Autodesk Inventor part; units mm, degrees
ref_plane "Work Plane1" through (-210, 0.3, -39.7) normal (1, 0, 0) x (0, 0, -1)
ref_plane "YZ Plane" through (0, 0, 0) normal (1, 0, 0) x (0, 1, 0)
ref_plane "XZ Plane" through (0, 0, 0) normal (0, 1, 0) x (-1, 0, 0)
sketch "Sketch1" plane through (0, 0, 0) normal (0, 1, 0) x (-1, 0, 0)
  line L0 (0, 0) -> (420, 0)
  line L1 (420, 0) -> (420, -40)
  line L2 (420, -40) -> (0, -40)
  line L3 (0, -40) -> (0, 0)
  dimension "d0" = 420
  dimension "d1" = 40
extrude "Extrusion1" add sketch "Sketch1" along normal blind 3.5
fillet "Fillet1" radius 0.3 10 edges at (-210, 3.5, 0) (-210, 0, 0) (0, 0, -20) (0, 3.5, -20) (0, 1.75, -40) (-210, 3.5, -40) (-210, 0, -40) (-420, 0, -20) (-420, 1.75, -40) (-420, 3.5, -20)
sketch "Sketch2" plane through (0, 0, 0) normal (0, -1, 0) x (1, 0, 0)
  line L0 (-419.7, -39.7) -> (-419.7, -0.3)
  line L1 (-419.7, -20) -> (0, -20)
  circle A0 centre (-405, -20) radius 5
  circle A1 centre (-375, -20) radius 5
  circle A2 centre (-345, -20) radius 5
  circle A3 centre (-315, -20) radius 5
  line L2 (-420, 0) -> (-420, -39.7)
  line L3 (-315, -20) -> (-315, -8.0411)
  line L4 (-210.3, -20) -> (-630, -20)
  circle A4 centre (-225, -20) radius 5
  circle A5 centre (-255, -20) radius 5
  circle A6 centre (-285, -20) radius 5
  point P0 (0, 0)
  point P1 (-420, -0.3)
  dimension "d5" = 10
  dimension "d6" = 10
  dimension "d7" = 10
  dimension "d8" = 10
  dimension "d9" = 15
  dimension "d10" = 30
  dimension "d11" = 30
  dimension "d12" = 30
ref_plane "Work Plane1" through (-210, 0.3, -39.7) normal (1, 0, 0) x (0, 0, -1)
extrude "Extrusion2" cut sketch "Sketch2" against normal blind 3
mirror "Mirror1" about plane through (-210, 0.3, -39.7) normal (1, 0, 0) of "Extrusion2"
fillet "Fillet2" radius 2 6 edges at (-0.0879, 3.4121, -0.0879) (-0.0879, 0.0879, -0.0879) (0, 1.75, 0) (-419.9121, 3.4121, -0.0879) (-419.9121, 0.0879, -0.0879) (-420, 1.75, 0)
sketch "Sketch3" plane through (0, 3.5, 0) normal (0, 1, 0) x (1, 0, 0)
  line L0 (4.2695, -58.2258) -> (-175.7305, -58.2258)
  line L1 (-175.7305, -58.2258) -> (-175.7305, 85.9661)
  line L2 (-175.7305, 85.9661) -> (4.2695, 85.9661)
  line L3 (4.2695, 85.9661) -> (4.2695, -58.2258)
  line L4 (-175.7305, 85.9661) -> (-355.7305, 85.9661)
  line L5 (-355.7305, 85.9661) -> (-355.7305, -58.2258)
  line L6 (-355.7305, -58.2258) -> (-175.7305, -58.2258)
  line L7 (-175.7305, -58.2258) -> (-175.7305, 85.9661)
  line L8 (-355.7305, -58.2258) -> (-453.8172, -58.2258)
  line L9 (-453.8172, -58.2258) -> (-453.8172, 85.9661)
  line L10 (-453.8172, 85.9661) -> (-355.7305, 85.9661)
  line L11 (-355.7305, 85.9661) -> (-355.7305, -58.2258)
  point P0 (0, 0)
  dimension "d18" = 180
  dimension "d19" = 180
extrude "Extrusion8" cut sketch "Sketch3" against normal through all contours L0 L1 L2 L3 | L6 L5 L4 L1
sketch "Sketch7" plane through (-355.7305, 3.5, -0.3) normal (1, 0, 0) x (0, 0, -1)
  line L0 (4.7, -1.75) -> (14.7, -1.75) construction
  line L1 (-0.3, -3.2) -> (-0.3, -0.3)
  line L2 (4.7, -2.5) -> (14.7, -2.5)
  line L3 (14.7, -1) -> (4.7, -1)
  arc A0 (4.7, -1) -> (4.7, -2.5) centre (4.7, -1.75) ccw
  arc A1 (14.7, -2.5) -> (14.7, -1) centre (14.7, -1.75) ccw
  line L4 (24.7, -1.75) -> (34.7, -1.75) construction
  line L5 (24.7, -2.5) -> (34.7, -2.5)
  line L6 (34.7, -1) -> (24.7, -1)
  arc A2 (24.7, -1) -> (24.7, -2.5) centre (24.7, -1.75) ccw
  arc A3 (34.7, -2.5) -> (34.7, -1) centre (34.7, -1.75) ccw
  line L7 (39.7, -0.3) -> (39.7, -3.2)
  point P0 (-0.3, -3.5)
  point P1 (9.7, -1.75)
  point P2 (29.7, -1.75)
  dimension "d56" = 5
  dimension "d57" = 1.5
  dimension "d58" = 5
  dimension "d59" = 1.5
  dimension "d60" = 10
  dimension "d61" = 10
extrude "Extrusion9" cut sketch "Sketch7" against normal blind 16
chamfer "Chamfer3" distance 0.3 angle 45 8 edges at (-355.7305, 2.5, -10) (-355.7305, 1.75, -15.75) (-355.7305, 1, -10) (-355.7305, 1.75, -4.25) (-355.7305, 1.75, -24.25) (-355.7305, 2.5, -30) (-355.7305, 1.75, -35.75) (-355.7305, 1, -30)
properties part number "LeftClamo3"
Read the model definition and answer for the solid it produces. Units are mm, in the model's axes. A direction names the side the tool comes from. Round coordinates to 2 decimals unless told otherwise and drop trailing zeros. Write each loop counter-clockwise with the first axis right and the second up, starting at its lowest first coordinate (ties: lowest second). Pieces come first, ordered by that corner, then holes. Notation, with made-up numbers: (4.5, 0.25) - (21.5, 0.25) arc R26 ccw to (21.5, 35.25) - close; hole circle Ø1 at (9.25, -37.75). An arc over 180 degrees is marked (long way). Use CSV: the item, a comma, the result in double quotes.
Q1. Each of these flat-tipped pins is pushed along its axis until it touches: pin 1 Ø3 at (x, z) = (-373.5, -18) entering from -Y; pin 2 Ø0.8 at (y, z) = (1.5, -8) entering from +X. Where does it stop, or does it pass through?
Values:
pin 1,"stops at y = 3"
pin 2,"stops at x = -371.73"
Q2. Straight lines are drawn through the part: line 1 along X through (y, z) = (1.6, -20); line 2 along Z through (x, y) = (-364.5, 1.75); line 3 along Z through (x, y) = (-405, 2.35). For each, find the intervals that lie inside material, in ascending order.
Values:
line 1,"x = -420 to -410, -400 to -380, -370 to -355.73"
line 2,"z = -40 to -35.75, -24.25 to -15.75, -4.25 to 0"
line 3,"z = -40 to -25, -15 to 0"
Q3. Find section A-A, the plane y = 1.75. Write down the section's boundary in (x, z).
Values:
outline,"(-420, -39.7) arc R0.3 ccw to (-419.7, -40) - (-355.73, -40) - (-355.73, -36.05) - (-356.03, -35.75) - (-371.73, -35.75) - (-371.73, -24.25) - (-356.03, -24.25) - (-355.73, -23.95) - (-355.73, -16.05) - (-356.03, -15.75) - (-371.73, -15.75) - (-371.73, -4.25) - (-356.03, -4.25) - (-355.73, -3.95) - (-355.73, 0) - (-418, 0) arc R2 ccw to (-420, -2) - close; hole circle Ø10 at (-405, -20); hole circle Ø10 at (-375, -20)"
Q4. A tool of negligible diameter and unlimited length cuts with its end or side. For faces 1 (the cylindrical face through (-400.381, 1.479, -21.915)), 2 (the flat face through (-364, 1, -30)), 3 (the flat face through (-388, 2, -40)), from which of +Z, -Z, +X, -X, +Y, -Y can it reach the whole face along a straight path? Write none if from no direction.
Values:
face 1,"-Y"
face 2,"+X"
face 3,"-Z, +X, -X, +Y, -Y"
Q5. Find section D-D, the plane x = -366.5. Write down the section's boundary in (y, z), then the cut area to 3 significant figures.
Values:
outline,"(0, -39.7) arc R0.3 ccw to (0.3, -40) - (3.2, -40) arc R0.3 ccw to (3.5, -39.7) - (3.5, -0.3) arc R0.3 ccw to (3.2, 0) - (0.3, 0) arc R0.3 ccw to (0, -0.3) - close; hole (1, -35) arc R0.75 ccw to (2.5, -35) - (2.5, -25) arc R0.75 ccw to (1, -25) - close; hole (1, -15) arc R0.75 ccw to (2.5, -15) - (2.5, -5) arc R0.75 ccw to (1, -5) - close"
area,"106 mm²"
Q6. Find section B-B, the plane x = -375. Write down the section's boundary in (y, z), then the cut area to 3 significant figures.
Values:
outline,"(0, -39.7) arc R0.3 ccw to (0.3, -40) - (3.2, -40) arc R0.3 ccw to (3.5, -39.7) - (3.5, -0.3) arc R0.3 ccw to (3.2, 0) - (0.3, 0) arc R0.3 ccw to (0, -0.3) - (0, -15) - (3, -15) - (3, -25) - (0, -25) - close"
area,"110 mm²"
Q7. Determine the mould class of faces 4 (the flat face through (-364, 1, -10)), 5 (the flat face through (-375, 3, -20)), 6 (the cylindrical face through (-363.77, 1.73, -15.75)), 7 (the cylindrical face through (-419.4, 1.73, -0.57)) for opening direction Y: +Y half, -Y half, draft (parallel to the pull), parting line (faces both ways), or undercut.
Values:
face 4,"undercut"
face 5,"-Y half"
face 6,"undercut"
face 7,"draft"
Q8. Find section C-C, the plane z = -32.5. Write down the section's boundary in (x, y), then the cut area to 3 significant figures.
Values:
outline,"(-420, 0.3) arc R0.3 ccw to (-419.7, 0) - (-355.73, 0) - (-355.73, 0.7) - (-356.03, 1) - (-371.73, 1) - (-371.73, 2.5) - (-356.03, 2.5) - (-355.73, 2.8) - (-355.73, 3.5) - (-419.7, 3.5) arc R0.3 ccw to (-420, 3.2) - close"
area,"201 mm²"
